from build123d import *

# Parameters (mm, degrees)
CUT_EXTRUDE1_DEPTH  = 6
SKETCH3_R           = 27.5
BOSS_EXTRUDE1_DEPTH = 63
CHAMFER1_SIZE       = 1
CUT_EXTRUDE2_DEPTH  = 6


with BuildPart() as part:
    # Sketch1 → Revolve1 (revolve)
    with BuildSketch(Plane.XY, mode=Mode.PRIVATE) as revolve1_sk:
        Polygon((-59.649564477, 0), (-59.649564477, 27.5), (-30.659969427, 27.5), (-30.659969427, 29.5), (35.33203125, 29.5), (35.33203125, 33.5), (36.33203125, 34.5), (40.340030573, 34.5), (41.340030573, 33.5), (41.340030573, 27.5), (69.340030573, 27.5), (70.340030573, 26.5), (70.340030573, 0), align=None)
    revolve(revolve1_sk.sketch.rotate(Axis((-72.236328125, 0, 0), (1, 0, 0)), 90), axis=Axis((-72.236328125, 0, 0), (1, 0, 0)))

    # Sketch2 → Cut-Extrude1 (cut)
    with BuildSketch(Plane(origin=(0, 29.5, 0), x_dir=(1, 0, 0), z_dir=(0, 1, 0))):
        with BuildLine():
            Line((-10.16796875, 8), (14.83203125, 8))
            ThreePointArc((14.83203125, 8), (22.83203125, 0), (14.83203125, -8))
            Line((14.83203125, -8), (-10.16796875, -8))
            ThreePointArc((-10.16796875, -8), (-18.16796875, 0), (-10.16796875, 8))
        make_face()
    extrude(amount=-CUT_EXTRUDE1_DEPTH, mode=Mode.SUBTRACT)

    # Sketch3 → Boss-Extrude1 (add)
    with BuildSketch(Plane.ZY.offset(59.649564477)):
        Circle(SKETCH3_R)
    extrude(amount=BOSS_EXTRUDE1_DEPTH)

    # Chamfer1
    chamfer1_edges = [part.edges().sort_by_distance(p)[0] for p in [
        (-122.649564477, 0, -27.5),
    ]]
    chamfer(chamfer1_edges, length=CHAMFER1_SIZE)

    # Sketch4 → Cut-Extrude2 (cut)
    with BuildSketch(Plane(origin=(0, 27.5, 0), x_dir=(1, 0, 0), z_dir=(0, 1, 0))):
        with BuildLine():
            Line((-102.649564477, 8), (-77.649564477, 8))
            ThreePointArc((-77.649564477, 8), (-69.649564477, 0), (-77.649564477, -8))
            Line((-77.649564477, -8), (-102.649564477, -8))
            ThreePointArc((-102.649564477, -8), (-110.649564477, 0), (-102.649564477, 8))
        make_face()
    extrude(amount=-CUT_EXTRUDE2_DEPTH, mode=Mode.SUBTRACT)


solid = part.part
Verification items for the finished model (mm, model axes). A direction names the side the tool comes from. Round coordinates to 2 decimals unless told otherwise and drop trailing zeros. Order: outer loops, then holes, each group sorted by start corner. A loop starts at its lowest first (then second) coordinate and runs counter-clockwise, first axis right, second up. Notation, with made-up numbers: (89.5, 4.25) -> (93.5, 4.25) arc R24 cw to (93.5, 36.25) -> close; hole circle Ø1 at (-22, 6.5). An arc over 180 degrees is marked (long way). Put each result on its own line as item: value.
1) Material ranges on line 1 (Y direction, x = 18, z = 1); line 2 (X direction, y = 15.5, z = -24.5); line 3 (Y direction, x = -84.5, z = 0), recorded low to high.
Final values:
line 1: y = -29.48 to 23.5
line 2: x = -30.66 to 41.34
line 3: y = -27.5 to 21.5
2) Mould release check, pull along X, two halves, no side actions. Record for faces 1 (the cylindrical face through (38.364, -1.517, -34.467)), 2 (the flat face through (-30.66, 20, -20)), 3 (the flat face through (3, 26, 8)): +X half, -X half, draft (parallel to the pull), parting line (faces both ways), or undercut.
Final values:
face 1: draft
face 2: -X half
face 3: undercut
3) Section check C-C (x = -96). Record the cut outline in (y, z).
Final values:
outline: (21.5, -8) -> (21.5, 8) -> (26.31, 8) arc R27.5 ccw (long way) to (26.31, -8) -> close
4) Section check B-B (y = 0). Record the cut outline in (x, z).
Final values:
outline: (-122.65, -26.5) -> (-121.65, -27.5) -> (-30.66, -27.5) -> (-30.66, -29.5) -> (35.33, -29.5) -> (35.33, -33.5) -> (36.33, -34.5) -> (40.34, -34.5) -> (41.34, -33.5) -> (41.34, -27.5) -> (69.34, -27.5) -> (70.34, -26.5) -> (70.34, 26.5) -> (69.34, 27.5) -> (41.34, 27.5) -> (41.34, 33.5) -> (40.34, 34.5) -> (36.33, 34.5) -> (35.33, 33.5) -> (35.33, 29.5) -> (-30.66, 29.5) -> (-30.66, 27.5) -> (-121.65, 27.5) -> (-122.65, 26.5) -> close
5) Depth check by flat-ended pin: pin 1 (1.4 mm diameter, centred on x = -93.5, y = 24.5, fed in from +Z); pin 2 (8 mm diameter, centred on x = 9, z = 2, fed in from +Y); pin 3 (17.5 mm diameter, centred on x = -99.5, z = 2.5, fed in from +Y). Enter the tip coordinate at first touch or a pass-through.
Final values:
pin 1: stops at z = 13.78
pin 2: stops at y = 23.5
pin 3: stops at y = 26.71
6) Set-up check for faces 4 (the cylindrical face through (55.536, 24.397, 12.69)), 5 (the cylindrical face through (2.8, -29.25, -3.84)), 6 (the flat face through (-90, 24, -8)): record each of +Z, -Z, +X, -X, +Y, -Y from which the full face is reachable in a straight line by a thin tool's end or side.
Final values:
face 4: +X
face 5: -X
face 6: +Y
7) Section check D-D (x = 29). Record the cut outline in (y, z).
Final values:
outline: circle Ø59 at (0, 0)
